```python
from build123d import *

# Parameters (mm, degrees)
BOSS_EXTRUDE1_DEPTH = 100
SKETCH2_R           = 1
CUT_EXTRUDE1_DEPTH  = 106.475115549


with BuildPart() as part:
    # Sketch1 → Boss-Extrude1 (new body)
    with BuildSketch(Plane(origin=(0, 0, 0), x_dir=(1, 0, 0), z_dir=(0, 1, 0))):
        with BuildLine():
            Line((15, -15), (-15, -15))
            ThreePointArc((-15, -15), (-30, 0), (-15, 15))
            Line((-15, 15), (15, 15))
            ThreePointArc((15, 15), (30, 0), (15, -15))
        make_face()
    extrude(amount=BOSS_EXTRUDE1_DEPTH)

    # Sketch2 → Cut-Extrude1 (cut, through all)
    with BuildSketch(Plane(origin=(0, 100, 0), x_dir=(1, 0, 0), z_dir=(0, 1, 0))):
        with Locations((-21.982299004, 13.275823915)):
            Circle(SKETCH2_R)
        with Locations((-30, 0)):
            Circle(SKETCH2_R)
        with Locations((-21.982299004, -13.275823915)):
            Circle(SKETCH2_R)
        with Locations((-27.321975393, 8.55388347)):
            Circle(SKETCH2_R)
        with Locations((-27.321975393, -8.55388347)):
            Circle(SKETCH2_R)
        with Locations((21.982299004, -13.275823915)):
            Circle(SKETCH2_R)
        with Locations((27.321975393, -8.55388347)):
            Circle(SKETCH2_R)
        with Locations((30, 0)):
            Circle(SKETCH2_R)
        with Locations((27.321975393, 8.55388347)):
            Circle(SKETCH2_R)
        with Locations((21.982299004, 13.275823915)):
            Circle(SKETCH2_R)
    extrude(amount=-CUT_EXTRUDE1_DEPTH, mode=Mode.SUBTRACT)


solid = part.part
```
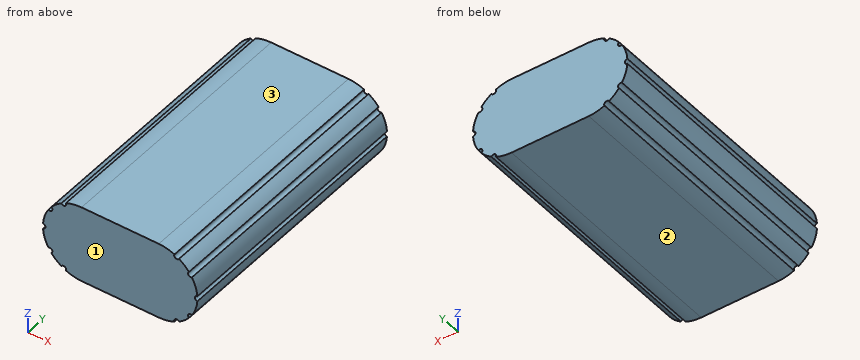
The model under review builds one solid part; all positions refer to its coordinate system, in mm. Face numbers are marked on the shaded views. Round coordinates to 2 decimals unless told otherwise and drop trailing zeros. Loops run counter-clockwise (first coordinate to the right, second up) from the corner with the lowest first, then second, coordinate; pieces in that order, holes last. Notation, with made-up numbers: (-33.75, -2) - (-8.75, -2) arc R16 cw to (-8.75, 18) - close; hole circle Ø9 at (45.5, 89). An arc over 180 degrees is marked (long way). Use a Markdown table: item, result. Add a question column.
Q1. The part is to be moulded in two halves that separate along Z. For the marked faces 1, 2 and 3, say which applies: pulls with the +Z half, pulls with the -Z half, needs draft (parallel to the pull), parting line crosses it, or undercut.
Q2. For probe 1 along X at (y, z) = (32.5, 9); probe 2 along Z at (x, y) = (-27, 89.5); probe 3 along X at (y, z) = (41, 11), list the stretches that pass through material, from the lowest coordinate up.
Q3. Add section B-B (z = 0). State the section outline as (x, y) points, plus the area to 3 significant figures.
Q4. Add section C-C (x = -19.5). State the section outline as (y, z) points, plus the area to 3 significant figures.
Q5. Add section A-A (y = 91). State the section outline as (x, z) points, plus the area to 3 significant figures.
Q6. Insertion check: pin 1 Ø10 at (x, y) = (22.5, 11) entering from -Z; pin 2 Ø6 at (y, z) = (24.5, -6.5) entering from -X; pin 3 Ø8 at (y, z) = (60.5, 6.5) entering from -X. Each pin has a flat end and moves straight along its axis. Give the tip position at first contact, or say it passes through.
Worked answers:
| question | item | result |
|---|---|---|
| 1 | face 1 | needs draft |
| 1 | face 2 | pulls with the -Z half |
| 1 | face 3 | pulls with the +Z half |
| 2 | probe 1 | -26.43 to 26.43 |
| 2 | probe 2 | -7.61 to 7.61 |
| 2 | probe 3 | -25.2 to 25.2 |
| 3 | outline | (-29, 0) - (29, 0) - (29, 100) - (-29, 100) - close |
| 3 | area | 5,800 mm² |
| 4 | outline | (0, -14.31) - (100, -14.31) - (100, 14.31) - (0, 14.31) - close |
| 4 | area | 2,860 mm² |
| 5 | outline | (-29.97, -1) arc R15 ccw to (-27.86, -7.71) arc R1 cw to (-26.72, -9.36) arc R15 ccw to (-22.85, -12.78) arc R1 cw to (-21.08, -13.71) arc R15 ccw to (-15, -15) - (15, -15) arc R15 ccw to (21.08, -13.71) arc R1 cw to (22.85, -12.78) arc R15 ccw to (26.72, -9.36) arc R1 cw to (27.86, -7.71) arc R15 ccw to (29.97, -1) arc R1 cw to (29.97, 1) arc R15 ccw to (27.86, 7.71) arc R1 cw to (26.72, 9.36) arc R15 ccw to (22.85, 12.78) arc R1 cw to (21.08, 13.71) arc R15 ccw to (15, 15) - (-15, 15) arc R15 ccw to (-21.08, 13.71) arc R1 cw to (-22.85, 12.78) arc R15 ccw to (-26.72, 9.36) arc R1 cw to (-27.86, 7.71) arc R15 ccw to (-29.97, 1) arc R1 cw to start |
| 5 | area | 1,590 mm² |
| 6 | pin 1 | z = -14.79 |
| 6 | pin 2 | x = -29.59 |
| 6 | pin 3 | x = -29.79 |
